Input: part model. Units: mm. Frame: model coordinates. A direction names the side the tool comes from. Coordinates: 2 decimals unless noted, no trailing zeros. Loops run counter-clockwise (first coordinate to the right, second up) from the corner with the lowest first, then second, coordinate; pieces in that order, holes last.
Item 1: Section C-C on x = -50. Return loops of the section in (y, z), and give its area (3 significant figures).
Item 2: Section D-D on y = -0.15. Give the number of separate pieces and of enclosed holes in the cut face, and give its area (3 significant figures).
Item 3: Section A-A on x = -109. Return loops of the section in (y, z), and give its area (3 significant figures).
Item 4: Reachability of faces 1 (the cylindrical face through (-57.682, -0.01, 4.746)), 2 (the cylindrical face through (-71, 0.01, 10.67)) from +Z, -Z, +X, -X, +Y, -Y: full face, straight path, thin tool, end or side. Return the list, or none.
Item 5: Pull-direction query (Z, two-part tool) for faces 3 (the cylindrical face through (-69.984, 0.01, -10.842)), 4 (the cylindrical face through (-33, 0, -20.8)), 5 (the cylindrical face through (-120, 0, 0)); classes: released by +Z, released by -Z, zero draft, split by the parting line, or undercut.
Item 6: Section B-B on z = 19.75. Return loops of the section in (x, y), and give its area (3 significant figures).
Item 7: Ray query, line 1 along X through (y, z) = (-0.05, 0); line 2 along Z through (x, y) = (-90, -0.6); line 3 along Z through (x, y) = (-115, 0). Return the intervals inside material, ascending.
```python
from build123d import *

# Parameters (mm, degrees)
SKETCH1_R                      = 3.5
BOSS_EXTRUDE1_DEPTH            = 0.75
F_2_2_2_2_DIAMETER_HOLE1_D     = 2.2
F_3_2_3_2_DIAMETER_HOLE1_D     = 3.2
F_3_2_3_2_DIAMETER_HOLE1_DEPTH = 10
F_3_2_3_2_DIAMETER_HOLE1_TIP   = 0.96137699
CUT_EXTRUDE1_DEPTH             = 2.5
FILLET1_R                      = 2
SKETCH7_R                      = 4
CUT_EXTRUDE2_DEPTH             = 2.5000001


with BuildPart() as part:
    # Sketch1 → Boss-Extrude1 (new body, symmetric)
    with BuildSketch(Plane(origin=(0, 0, 0), x_dir=(1, 0, 0), z_dir=(0, 1, 0))):
        with BuildLine():
            ThreePointArc((-37.239092363, -21.5), (-43, 0), (-37.239092363, 21.5))
            ThreePointArc((-37.239092363, 21.5), (-36.658838331, 22.248681329), (-35.899079455, 22.81435343))
            ThreePointArc((-35.899079455, 22.81435343), (-70.492179883, 10.7556392), (-107.126701642, 10.839315166))
            ThreePointArc((-107.126701642, 10.839315166), (-120, 0), (-107.126701642, -10.839315166))
            ThreePointArc((-107.126701642, -10.839315166), (-70.492179883, -10.7556392), (-35.899079455, -22.81435343))
            ThreePointArc((-35.899079455, -22.81435343), (-36.658838331, -22.248681329), (-37.239092363, -21.5))
        make_face()
        with BuildLine():
            ThreePointArc((-31.176914536, 18), (-35.958003449, 16.718911087), (-37.239092363, 21.5))
            ThreePointArc((-37.239092363, 21.5), (-43, 0), (-37.239092363, -21.5))
            ThreePointArc((-37.239092363, -21.5), (-35.958003449, -16.718911087), (-31.176914536, -18))
            ThreePointArc((-31.176914536, -18), (-36, 0), (-31.176914536, 18))
        make_face()
        with Locations((-34.208003449, -19.75)):
            Circle(SKETCH1_R)
        with Locations((-34.208003449, 19.75)):
            Circle(SKETCH1_R)
    extrude(amount=BOSS_EXTRUDE1_DEPTH, both=True)

    # Ø2.2 (2.2) Diameter Hole1 (through all)
    with Locations(Plane(origin=(0, 0.75, 0), x_dir=(1, 0, 0), z_dir=(0, 1, 0))):
        with Locations((-114.480077554, 5.480077554), (-103.519922446, 5.480077554), (-103.519922446, -5.480077554), (-114.480077554, -5.480077554)):
            Hole(F_2_2_2_2_DIAMETER_HOLE1_D / 2)

    # Ø3.2 (3.2) Diameter Hole1
    with Locations(Plane(origin=(0, 0.75, 0), x_dir=(1, 0, 0), z_dir=(0, 1, 0))):
        with Locations((-34.208003449, 19.75), (-34.208003449, -19.75), (-95.790276336, 5.979398024), (-95.790276336, -5.979398024)):
            Hole(F_3_2_3_2_DIAMETER_HOLE1_D / 2, depth=F_3_2_3_2_DIAMETER_HOLE1_DEPTH)
            with Locations((0, 0, -(F_3_2_3_2_DIAMETER_HOLE1_DEPTH + F_3_2_3_2_DIAMETER_HOLE1_TIP / 2))):  # 118° drill point
                Cone(0, F_3_2_3_2_DIAMETER_HOLE1_D / 2, F_3_2_3_2_DIAMETER_HOLE1_TIP, mode=Mode.SUBTRACT)

    # Sketch6 → Cut-Extrude1 (cut, through all)
    with BuildSketch(Plane(origin=(0, 0.75, 0), x_dir=(1, 0, 0), z_dir=(0, 1, 0))):
        with BuildLine():
            Line((-72.469338063, -3.369046694), (-49.802019621, 0))
            Line((-49.802019621, 0), (-72.469338063, 3.369046694))
            ThreePointArc((-72.469338063, 3.369046694), (-85.377857375, 2.290839769), (-98.326107181, 2.65857332))
            ThreePointArc((-98.326107181, 2.65857332), (-98, 0), (-98.326107181, -2.65857332))
            ThreePointArc((-98.326107181, -2.65857332), (-85.377857375, -2.290839769), (-72.469338063, -3.369046694))
        make_face()
        with BuildLine():
            Line((-66.096117167, 4.443764231), (-42.988154947, 1.009224591))
            ThreePointArc((-42.988154947, 1.009224591), (-42.467311238, 6.747405149), (-41.183985346, 12.36443897))
            ThreePointArc((-41.183985346, 12.36443897), (-53.416219701, 7.70010587), (-66.096117167, 4.443764231))
        make_face()
        with BuildLine():
            ThreePointArc((-41.183985346, -12.36443897), (-42.467311238, -6.747405149), (-42.988154947, -1.009224591))
            Line((-42.988154947, -1.009224591), (-66.096117167, -4.443764231))
            ThreePointArc((-66.096117167, -4.443764231), (-53.416219701, -7.70010587), (-41.183985346, -12.36443897))
        make_face()
    extrude(amount=-CUT_EXTRUDE1_DEPTH, mode=Mode.SUBTRACT)

    # Fillet1
    fillet1_edges = [part.edges().sort_by_distance(p)[0] for p in [
        (-42.988154947, 0, 1.009224591),
        (-41.183985346, 0, 12.36443897),
        (-66.096117167, 0, 4.443764231),
        (-98.326107181, 0, 2.65857332),
        (-98.326107181, 0, -2.65857332),
        (-72.469338063, 0, -3.369046694),
        (-49.802019621, 0, 0),
        (-72.469338063, 0, 3.369046694),
        (-41.183985346, 0, -12.36443897),
        (-42.988154947, 0, -1.009224591),
        (-66.096117167, 0, -4.443764231),
    ]]
    fillet(fillet1_edges, radius=FILLET1_R)

    # Sketch7 → Cut-Extrude2 (cut, through all)
    with BuildSketch(Plane(origin=(0, 0.75, 0), x_dir=(1, 0, 0), z_dir=(0, 1, 0))):
        with Locations((-109, 0)):
            Circle(SKETCH7_R)
    extrude(amount=-CUT_EXTRUDE2_DEPTH, mode=Mode.SUBTRACT)


solid = part.part
```
Results found:
1. outline: (-0.75, -16.3) - (0.75, -16.3) - (0.75, -8.84) - (-0.75, -8.84) - close; (-0.75, -2.05) - (0.75, -2.05) - (0.75, 2.05) - (-0.75, 2.05) - close; (-0.75, 8.84) - (0.75, 8.84) - (0.75, 16.3) - (-0.75, 16.3) - close
1. area: 28.5 mm2
2. separate pieces: 1
2. enclosed holes: 12
2. area: 1,650 mm2
3. outline: (-0.75, -11) - (0.75, -11) - (0.75, -4) - (-0.75, -4) - close; (-0.75, 4) - (0.75, 4) - (0.75, 11) - (-0.75, 11) - close
3. area: 21.0 mm2
4. face 1: +Y, -Y
4. face 2: +Z, +Y, -Y
5. face 3: released by -Z
5. face 4: undercut
5. face 5: split by the parting line
6. outline: (-41.88, -0.75) - (-35.81, -0.75) - (-35.81, 0.75) - (-41.88, 0.75) - close; (-32.61, -0.75) - (-30.71, -0.75) - (-30.71, 0.75) - (-32.61, 0.75) - close
6. area: 12.0 mm2
7. line 1: x = -120 to -113, -105 to -98, -61.41 to -36
7. line 2: z = -9.26 to -2.26, 2.26 to 9.26
7. line 3: z = -9.22 to -6.45, -4.51 to 4.51, 6.45 to 9.22
